Read the model definition and answer for the solid it produces. Units are mm, in the model's axes. A direction names the side the tool comes from. Give positions to 0.01 mm unless a question says otherwise; leave off trailing zeros. Write each loop counter-clockwise with the first axis right and the second up, starting at its lowest first coordinate (ties: lowest second). Pieces come first, ordered by that corner, then holes. Notation, with made-up numbers: (-30, 44) -> (22, 44) arc R38 cw to (22, 82) -> close; hole circle Ø11 at (32, 6). An arc over 180 degrees is marked (long way). Use a Markdown table: item, result.
Autodesk Inventor part; units mm, degrees
ref_plane "YZ Plane" through (0, 0, 0) normal (1, 0, 0) x (0, 1, 0)
ref_plane "XZ Plane" through (0, 0, 0) normal (0, 1, 0) x (-1, 0, 0)
ref_plane "XY Plane" through (0, 0, 0) normal (0, 0, 1) x (1, 0, 0)
sketch "Sketch1" plane through (0, 0, 0) normal (0, 1, 0) x (-1, 0, 0)
  circle A0 centre (0, 0) radius 6.35
  dimension "d0" = 0
  dimension "d1" = 0
  dimension "d2" = 12.7
extrude "Extrusion1" add sketch "Sketch1" along normal blind 127
sketch "Sketch2" plane through (0, 127, 0) normal (0, 1, 0) x (1, 0, 0)
  point P0 (0, 0)
  point P1 (0, 0)
hole "Hole1" at (0, 127, 0) direction (0, -1, 0) diameter 4.9784 depth 19.05 tip angle 118
sketch "Sketch3" plane through (0, 0, 0) normal (0, -1, 0) x (1, 0, 0)
  circle A0 centre (0, 0) radius 2.4892
hole "Hole2" at (0, 0, 0) direction (0, 1, 0) diameter 4.9784 depth 19.05 tip angle 118
properties part number "Short Support"
Item 1: A tool of negligible diameter and unlimited length cuts with its end or side. For faces 4 (the face through (-0.748, 9.658, -2.374)), 5 (the face through (-0.748, 117.342, 2.374)), 6 (the face through (-3, 0, 0)), from which of +Z, -Z, +X, -X, +Y, -Y can it reach the whole face along a straight path? Write none if from no direction.
Return value:
| item | result |
|---|---|
| face 4 | -Y |
| face 5 | +Y |
| face 6 | +Z, -Z, +X, -X, -Y |
Item 2: A cutting plane is placed at A-A (y = 69). Give the vertices of the cut face in (x, z), then the cut area to 3 significant figures.
Return value:
| item | result |
|---|---|
| outline | circle Ø12.7 at (0, 0) |
| area | 127 mm^2 |
Item 3: A cutting plane is placed at B-B (x = -5). Give the vertices of the cut face in (y, z).
Return value:
| item | result |
|---|---|
| outline | (0, -3.91) -> (127, -3.91) -> (127, 3.91) -> (0, 3.91) -> close |
Item 4: For a pull along X with two mould halves and no side action, classify faces 1 (the face through (-3, 127, 0)), 2 (the face through (-0.26, 106.71, -0.34)), 3 (the face through (1.38, 62.61, 6.2)) as +X half, -X half, draft (parallel to the pull), parting line (faces both ways), or undercut.
Return value:
| item | result |
|---|---|
| face 1 | draft |
| face 2 | undercut |
| face 3 | parting line |
Item 5: Straight lines are drawn through the part: line 1 along Z through (x, y) = (0, 13.5); line 2 along X through (y, z) = (110.5, -2); line 3 along Z through (x, y) = (-3.75, 8.5). For each, find the intervals that lie inside material, in ascending order. Write a range as [from, to].
Return value:
| item | result |
|---|---|
| line 1 | [-6.35, -2.49], [2.49, 6.35] |
| line 2 | [-6.03, -1.48], [1.48, 6.03] |
| line 3 | [-5.12, 5.12] |
Item 6: Each of these flat-tipped pins is pushed along its axis until it touches: P1, Ø2, axis at y = 75, z = 2, coming from the +X side; P2, Ø4, axis at y = 14.5, z = 4, coming from the +X side; P3, Ø6.5, axis at x = 0, z = 0, coming from the +Y side. Where does it stop, or does it pass through?
Return value:
| item | result |
|---|---|
| P1 | x = 6.27 |
| P2 | x = 6.03 |
| P3 | y = 127 |
